Geometry check sheet. Reference: the model listing, model coordinates, mm. Give positions to 0.01 mm unless a question says otherwise; leave off trailing zeros. Write each loop counter-clockwise with the first axis right and the second up, starting at its lowest first coordinate (ties: lowest second). Pieces come first, ordered by that corner, then holes. Notation, with made-up numbers: (46, 41) -> (71, 41) arc R13 cw to (71, 59) -> close; hole circle Ø2 at (15.25, 29.25). An arc over 180 degrees is marked (long way). Write item = value, one per line. Start each with the question number.
1. Depth check by flat-ended pin: P1, Ø0.8, axis at x = 48.5, y = -1, coming from the -Z side; P2, Ø0.5, axis at x = 48, y = -0.5, coming from the +Z side. Enter the tip coordinate at first touch or a pass-through.
2. Mould release check, pull along X, two halves, no side actions. Record for faces 1 (the flat face through (-1, -1.6, 0)), 2 (the cylindrical face through (-76.034, -0.789, 0.451)): pulls with the +X half, pulls with the -X half, needs draft (parallel to the pull), parting line crosses it, or undercut.
3. Cross-section at A-A, the plane y = -0.3. State how many separate pieces and enclosed holes the cut face has, plus the area to 3 significant figures.
4. Thickness scan on line 1 along X through (y, z) = (-0.9, -0.75); line 2 along X through (y, z) = (-1.2, -3.5); line 3 along X through (y, z) = (-0.6, -2.5). Record the ranges inside material, lowest first.
5. Cross-section at B-B, the plane x = -48. Record the cut outline in (y, z), plus the area to 3 significant figures.
```python
from build123d import *

# Parameters (mm, degrees)
F0_R     = 1.5
F1_DEPTH = 1.6


with BuildPart() as f1:
    # F0 (on Front) → F1 (new body)
    with BuildSketch(Plane.XZ):
        with BuildLine():
            Line((-45.73225, 8.25), (-49.73225, 8.25))
            Line((-49.73225, 8.25), (-49.73225, 10))
            Line((-49.73225, 10), (-93.4645, 10))
            Line((-93.4645, 10), (-93.4645, 5))
            Line((-93.4645, 5), (-87.4645, 5))
            ThreePointArc((-87.4645, 5), (-83.928966, 3.535534), (-82.4645, 0))
            ThreePointArc((-82.4645, 0), (-83.928966, -3.535534), (-87.4645, -5))
            Line((-87.4645, -5), (-93.4645, -5))
            Line((-93.4645, -5), (-93.4645, -10))
            Line((-93.4645, -10), (-49.73225, -10))
            Line((-49.73225, -10), (-49.73225, -8.25))
            Line((-49.73225, -8.25), (-45.73225, -8.25))
            Line((-45.73225, -8.25), (-45.73225, -10))
            Line((-45.73225, -10), (0, -10))
            Line((0, -10), (45.73225, -10))
            Line((45.73225, -10), (45.73225, -8.25))
            Line((45.73225, -8.25), (49.73225, -8.25))
            Line((49.73225, -8.25), (49.73225, -10))
            Line((49.73225, -10), (93.4645, -10))
            Line((93.4645, -10), (93.4645, -5))
            Line((93.4645, -5), (87.4645, -5))
            ThreePointArc((87.4645, -5), (83.928966, -3.535534), (82.4645, 0))
            ThreePointArc((82.4645, 0), (83.928966, 3.535534), (87.4645, 5))
            Line((87.4645, 5), (93.4645, 5))
            Line((93.4645, 5), (93.4645, 10))
            Line((93.4645, 10), (49.73225, 10))
            Line((49.73225, 10), (49.73225, 8.25))
            Line((49.73225, 8.25), (45.73225, 8.25))
            Line((45.73225, 8.25), (45.73225, 10))
            Line((45.73225, 10), (0, 10))
            Line((0, 10), (-45.73225, 10))
            Line((-45.73225, 10), (-45.73225, 8.25))
        make_face()
        with Locations((-77.4645, 0)):
            Circle(F0_R, mode=Mode.SUBTRACT)
        with Locations((77.4645, 0)):
            Circle(F0_R, mode=Mode.SUBTRACT)
    extrude(amount=F1_DEPTH)


solid = f1.part
```
Answers:
q1.P1 = -8.25
q1.P2 = 8.25
q2.face_1 = needs draft
q2.face_2 = undercut
q3.separate_pieces = 1
q3.enclosed_holes = 2
q3.area = 3,500 mm^2
q4.line_1 = -82.52 to -78.76, -76.17 to 76.17, 78.76 to 82.52
q4.line_2 = -83.89 to 83.89
q4.line_3 = -83.13 to 83.13
q5.outline = (-1.6, -8.25) -> (0, -8.25) -> (0, 8.25) -> (-1.6, 8.25) -> close
q5.area = 26.4 mm^2
